from build123d import *

# Parameters (mm, degrees)
CROQUIS1_R              = 1.6
CROQUIS1_R_2            = 1.528989044
CROQUIS1_R_3            = 1.814858399
SALIENTE_EXTRUIR1_DEPTH = 4.5
CROQUIS2_R              = 3.1
CROQUIS2_R_2            = 17
CORTAR_EXTRUIR1_DEPTH   = 5.5
CROQUIS3_R              = 2.75
CORTAR_EXTRUIR2_DEPTH   = 3
CROQUIS4_W              = 38
CROQUIS4_H              = 25
CROQUIS4_W_2            = 34.8
CROQUIS4_H_2            = 21.8
SALIENTE_EXTRUIR2_DEPTH = 82
CROQUIS5_R              = 1.6
CORTAR_EXTRUIR3_DEPTH   = 82
CORTAR_EXTRUIR4_REACH   = 116
CROQUIS6_R              = 4
REDONDEO1_R             = 2
REDONDEO2_R             = 1
CHAFL_N1_SIZE           = 0.5


with BuildPart() as part:
    # Croquis1 → Saliente-Extruir1 (new body)
    with BuildSketch(Plane(origin=(0, 0, 0), x_dir=(1, 0, 0), z_dir=(0, 1, 0))):
        Polygon((76, 25), (76, 0), (38, 0), (38, -25), (-38, -25), (-38, 0), (-38, 25), align=None)
        with Locations((-15, 21.5)):
            Circle(CROQUIS1_R, mode=Mode.SUBTRACT)
        with Locations((15, 21.5)):
            Circle(CROQUIS1_R, mode=Mode.SUBTRACT)
        with Locations((-23, -21.5)):
            Circle(CROQUIS1_R_2, mode=Mode.SUBTRACT)
        with Locations((23, -21.5)):
            Circle(CROQUIS1_R_3, mode=Mode.SUBTRACT)
        with Locations((61, 21.5)):
            Circle(CROQUIS1_R, mode=Mode.SUBTRACT)
    extrude(amount=SALIENTE_EXTRUIR1_DEPTH)

    # Croquis2 → Cortar-Extruir1 (cut, through all)
    with BuildSketch(Plane(origin=(0, 4.5, 0), x_dir=(1, 0, 0), z_dir=(0, 1, 0))):
        with Locations((29.5, 17.5)):
            Circle(CROQUIS2_R)
        with Locations((-5.5, -17.5)):
            Circle(CROQUIS2_R)
        with Locations((12, 0)):
            Circle(CROQUIS2_R_2)
    extrude(amount=-CORTAR_EXTRUIR1_DEPTH, mode=Mode.SUBTRACT)

    # Croquis3 → Cortar-Extruir2 (cut)
    with BuildSketch(Plane(origin=(0, 4.5, 0), x_dir=(1, 0, 0), z_dir=(0, 1, 0))):
        with Locations((-15, 21.5)):
            Circle(CROQUIS3_R)
        with Locations((15, 21.5)):
            Circle(CROQUIS3_R)
        with Locations((61, 21.5)):
            Circle(CROQUIS3_R)
        with Locations((23, -21.5)):
            Circle(CROQUIS3_R)
        with Locations((-23, -21.5)):
            Circle(CROQUIS3_R)
    extrude(amount=-CORTAR_EXTRUIR2_DEPTH, mode=Mode.SUBTRACT)

    # Croquis4 → Saliente-Extruir2 (add)
    with BuildSketch(Plane(origin=(0, 4.5, 0), x_dir=(1, 0, 0), z_dir=(0, 1, 0))):
        with Locations((57, -12.5)):
            Rectangle(CROQUIS4_W, CROQUIS4_H)
        with Locations((57, -12.5)):
            Rectangle(CROQUIS4_W_2, CROQUIS4_H_2, mode=Mode.SUBTRACT)
    extrude(amount=-SALIENTE_EXTRUIR2_DEPTH)

    # Croquis5 → Cortar-Extruir3 (cut)
    with BuildSketch(Plane.XY.offset(1.6)):
        with Locations((53.5, -73.5)):
            Circle(CROQUIS5_R)
    extrude(amount=-CORTAR_EXTRUIR3_DEPTH, mode=Mode.SUBTRACT)

    # Croquis6 → Cortar-Extruir4 (cut, up to next)
    with BuildSketch(Plane(origin=(76, 0, 0), x_dir=(0, 0, -1), z_dir=(1, 0, 0)), mode=Mode.PRIVATE) as cortar_extruir4_sk1:
        with Locations((-8.049586481, -34.845975381)):
            Circle(CROQUIS6_R)
    cortar_extruir4_tool1 = extrude(cortar_extruir4_sk1.sketch, amount=-CORTAR_EXTRUIR4_REACH, mode=Mode.PRIVATE) & part.part
    add(cortar_extruir4_tool1.solids().sort_by_distance((76, -34.845975, 8.049586))[0], mode=Mode.SUBTRACT)

    # Redondeo1
    redondeo1_edges = [part.edges().sort_by_distance(p)[0] for p in [
        (-38, 2.25, 25),
        (-38, 2.25, -25),
        (76, 2.25, -25),
        (76, -36.5, 25),
    ]]
    fillet(redondeo1_edges, radius=REDONDEO1_R)

    # Redondeo2
    redondeo2_edges = [part.edges().sort_by_distance(p)[0] for p in [
        (74.4, -36.5, 23.4),
    ]]
    fillet(redondeo2_edges, radius=REDONDEO2_R)

    # Chaflán1
    chafl_n1_edges = [part.edges().sort_by_distance(p)[0] for p in [
        (76, -77.5, 11.5),
        (75.414213562, -77.5, 24.414213562),
        (56, -77.5, 25),
    ]]
    chamfer(chafl_n1_edges, length=CHAFL_N1_SIZE)


solid = part.part
For this review, take the finished solid that the model builds, in its own axes (mm). A direction names the side the tool comes from. Round coordinates to 2 decimals unless told otherwise and drop trailing zeros. Write each loop counter-clockwise with the first axis right and the second up, starting at its lowest first coordinate (ties: lowest second). Pieces come first, ordered by that corner, then holes. Notation, with made-up numbers: (-39.75, -28) - (-22.75, -28) arc R17 ccw to (-22.75, 3) - close; hole circle Ø7 at (59, -19.5). An arc over 180 degrees is marked (long way). Use a Markdown table: item, result.
Q1. Wall thickness on line 1 along X through (y, z) = (0.5, -21.5); line 2 along X through (y, z) = (2.8, 21.5); line 3 along X through (y, z) = (-73.5, 1): over which ranges is each line inside the solid? List them lowest first.
Derived:
| item | result |
|---|---|
| line 1 | x = -38 to -16.6, -13.4 to 13.4, 16.6 to 59.4, 62.6 to 76 |
| line 2 | x = -38 to -25.75, -20.25 to 20.25, 25.75 to 39.6, 74.4 to 76 |
| line 3 | x = 38 to 51.9, 55.1 to 76 |
Q2. Machinability: for faces 5 (the flat face through (57, -38, 0)), 6 (the flat face through (57, -36, 1.6)), 7 (the cylindrical face through (54.36, -72.15, 0.81)), 8 (the flat face through (-22, 1.5, 23)), which of the approach directions +Z, -Z, +X, -X, +Y, -Y give a long, thin tool a straight path to every point of the face, cutting with its end or side? Answer none if there is none.
Derived:
| item | result |
|---|---|
| face 5 | -Z, +X, -X, -Y |
| face 6 | +Y, -Y |
| face 7 | -Z |
| face 8 | +Y |
Q3. We need section C-C (y = -27). Give the boundary of the cut face in (x, z).
Derived:
| item | result |
|---|---|
| outline | (38, 0) - (76, 0) - (76, 23) arc R2 ccw to (74, 25) - (38, 25) - close; hole (39.6, 1.6) - (74.4, 1.6) - (74.4, 22.4) arc R1 ccw to (73.4, 23.4) - (39.6, 23.4) - close |
Q4. We need section B-B (x = 61). Give the boundary of the cut face in (y, z), plus the area to 3 significant figures.
Derived:
| item | result |
|---|---|
| outline | (-77.5, 0) - (0, 0) - (0, -19.9) - (1.5, -19.9) - (1.5, -18.75) - (4.5, -18.75) - (4.5, 1.6) - (-77.5, 1.6) - close; (-77.5, 23.4) - (4.5, 23.4) - (4.5, 25) - (-77, 25) - (-77.5, 24.5) - close; (0, -25) - (4.5, -25) - (4.5, -24.25) - (1.5, -24.25) - (1.5, -23.1) - (0, -23.1) - close |
| area | 353 mm2 |
Q5. The part is to be moulded in two halves that separate along X. For faces 1 (the flat face through (74.4, -35.9, 12.1)), 2 (the flat face through (7, 0, -17)), 3 (the flat face through (38, -38, 13)), 4 (the flat face through (76, -37, 15)), say which applies: pulls with the +X half, pulls with the -X half, needs draft (parallel to the pull), parting line crosses it, or undercut.
Derived:
| item | result |
|---|---|
| face 1 | undercut |
| face 2 | needs draft |
| face 3 | pulls with the -X half |
| face 4 | pulls with the +X half |
Q6. We need section D-D (z = -4.5). Give the boundary of the cut face in (x, y), plus the area to 3 significant figures.
Derived:
| item | result |
|---|---|
| outline | (-38, 0) - (-4.39, 0) - (-4.39, 4.5) - (-38, 4.5) - close; (28.39, 0) - (76, 0) - (76, 4.5) - (28.39, 4.5) - close |
| area | 365 mm2 |
Q7. Clearance check with flat-ended pins moving along their axes: pin 1 (1.6 mm diameter, centred on x = 60, z = -21.5, fed in from +Y); pin 2 (3 mm diameter, centred on x = -15, z = -21.5, fed in from +Y); pin 3 (7 mm diameter, centred on x = 29.5, z = -17.5, fed in from -Y); pin 4 (12.5 mm diameter, centred on y = -41.5, z = 9, fed in from -X). State where each tip first meets the part, or that it passes through.
Derived:
| item | result |
|---|---|
| pin 1 | stops at y = 1.5 |
| pin 2 | passes through |
| pin 3 | stops at y = 0 |
| pin 4 | stops at x = 38 |
Q8. We need section A-A (x = 41). Give the boundary of the cut face in (y, z), plus the area to 3 significant figures.
Derived:
| item | result |
|---|---|
| outline | (-77.5, 0) - (0, 0) - (0, -25) - (4.5, -25) - (4.5, 1.6) - (-77.5, 1.6) - close; (-77.5, 23.4) - (4.5, 23.4) - (4.5, 25) - (-77, 25) - (-77.5, 24.5) - close |
| area | 375 mm2 |
